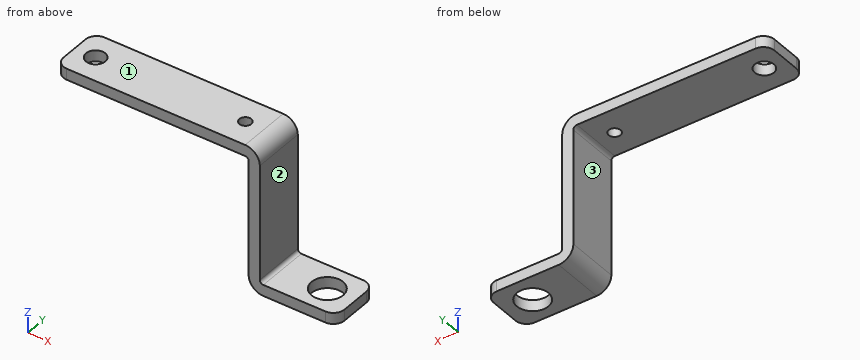
```python
from build123d import *

# Parameters (mm, degrees)
BASE_FLANGE1_DEPTH   = 3.175
EDGE_FLANGE1_DEPTH   = 15
EDGE_FLANGE2_DEPTH   = 15
M5_CLEARANCE_HOLE1_D = 5.5
M8_CLEARANCE_HOLE1_D = 9
FILLET1_R            = 3.175
M3_CLEARANCE_HOLE1_D = 3.4


# Sheet-metal steps are written as plain solids
with BuildPart() as part:
    # Sketch2 → Base-Flange1 (new body)
    with BuildSketch(Plane.XY):
        Polygon((79.909284585, 306.128054742), (73.909284585, 306.128054742), (73.909284585, 321.128054742), (79.909284585, 321.128054742), (127.909284585, 321.128054742), (127.909284585, 306.128054742), align=None)
    extrude(amount=BASE_FLANGE1_DEPTH)

    # Edge-Flange1 section (across the edge) → Edge-Flange1 (add)
    with BuildSketch(Plane(origin=(128.909284585, 321.128054742, 0), x_dir=(-1, 0, 0), z_dir=(0, -1, 0))):
        with BuildLine():
            Line((-3.175, 1), (-3.175, 33.738))
            Line((-3.175, 33.738), (0, 33.738))
            Line((0, 33.738), (0, 1))
            ThreePointArc((0, 1), (0.292893219, 0.292893219), (1, 0))
            Line((1, 0), (1, -3.175))
            ThreePointArc((1, -3.175), (-1.952170811, -1.952170811), (-3.175, 1))
        make_face()
    extrude(amount=EDGE_FLANGE1_DEPTH)

    # Edge-Flange2 section (across the edge) → Edge-Flange2 (add)
    with BuildSketch(Plane(origin=(132.084284585, 306.128054742, -34.738), x_dir=(0, 0, 1), z_dir=(0, 1, 0))):
        with BuildLine():
            Line((-3.175, 1), (-3.175, 21.825))
            Line((-3.175, 21.825), (0, 21.825))
            Line((0, 21.825), (0, 1))
            ThreePointArc((0, 1), (0.292893219, 0.292893219), (1, 0))
            Line((1, 0), (1, -3.175))
            ThreePointArc((1, -3.175), (-1.952170811, -1.952170811), (-3.175, 1))
        make_face()
    extrude(amount=EDGE_FLANGE2_DEPTH)

    # M5 Clearance Hole1 (through all)
    with Locations(Plane.XY.offset(3.175)):
        with Locations((79.909284585, 313.628054742)):
            Hole(M5_CLEARANCE_HOLE1_D / 2)

    # M8 Clearance Hole1 (through all)
    with Locations(Plane.XY.offset(-34.738)):
        with Locations((145.909284585, 313.628054742)):
            Hole(M8_CLEARANCE_HOLE1_D / 2)

    # Fillet1
    fillet1_edges = [part.edges().sort_by_distance(p)[0] for p in [
        (73.909284585, 306.128054742, 1.5875),
        (73.909284585, 321.128054742, 1.5875),
        (153.909284585, 306.128054742, -36.3255),
        (153.909284585, 321.128054742, -36.3255),
    ]]
    fillet(fillet1_edges, radius=FILLET1_R)

    # M3 Clearance Hole1 (through all)
    with Locations(Plane.XY.offset(3.175)):
        with Locations((122.609284585, 313.578054742)):
            Hole(M3_CLEARANCE_HOLE1_D / 2)


solid = part.part
```
The model under review builds one solid part; all positions refer to its coordinate system, in mm. Face numbers are marked on the shaded views. A direction names the side the tool comes from. Round coordinates to 2 decimals unless told otherwise and drop trailing zeros. Write each loop counter-clockwise with the first axis right and the second up, starting at its lowest first coordinate (ties: lowest second). Pieces come first, ordered by that corner, then holes. Notation, with made-up numbers: (-13, 88.25) -> (9, 88.25) arc R30 cw to (9, 122.25) -> close; hole circle Ø6 at (68, -38.5). An arc over 180 degrees is marked (long way). Use CSV: the item, a comma, the result in double quotes.
Q1. Consider section A-A (x = 148). Give the boundary of the cut face in (y, z), then the cut area to 3 significant figures.
Checks:
outline,"(306.13, -37.91) -> (309.64, -37.91) -> (309.64, -34.74) -> (306.13, -34.74) -> close; (317.61, -37.91) -> (321.13, -37.91) -> (321.13, -34.74) -> (317.61, -34.74) -> close"
area,"22.3 mm²"
Q2. Consider section B-B (y = 308). Give the boundary of the cut face in (x, z) (3 decimals), then the cut area to 3 significant figures.
Checks:
outline,"(74.189, 0) -> (127.909, 0) arc R1 cw to (128.909, -1) -> (128.909, -33.738) arc R4.175 ccw to (133.084, -37.913) -> (153.63, -37.913) -> (153.63, -34.738) -> (133.084, -34.738) arc R1 cw to (132.084, -33.738) -> (132.084, -1) arc R4.175 ccw to (127.909, 3.175) -> (74.189, 3.175) -> close"
area,"366 mm²"
Q3. For pin 1 Ø2 at (x, y) = (96.5, 311.5) entering from -Z; pin 2 Ø4.5 at (y, z) = (315, -17.5) entering from +X; pin 3 Ø1.5 at (y, z) = (310, -19.5) entering from -X; pin 4 Ø4.5 at (x, y) = (79.91, 313.63) entering from +Z, all flat-tipped, find the tip position at first contact; note any pin that passes through.
Checks:
pin 1,"z = 0"
pin 2,"x = 132.08"
pin 3,"x = 128.91"
pin 4,"through"
Q4. For the marked faces 1, 2 and 3, list the 3-axis set-ups (+Z, -Z, +X, -X, +Y, -Y) from which the entire face can be reached by the end or side of a thin tool; tool diameter is ignored.
Checks:
face 1,"+Z, +X, -X, +Y, -Y"
face 2,"+Z, +X, +Y, -Y"
face 3,"-Z, -X, +Y, -Y"
Q5. Consider section C-C (z = -30.5). Give the boundary of the cut face in (x, y).
Checks:
outline,"(128.91, 306.13) -> (132.08, 306.13) -> (132.08, 321.13) -> (128.91, 321.13) -> close"
Q6. Consider section D-D (x = 138.5). Give the boundary of the cut face in (y, z).
Checks:
outline,"(306.13, -37.91) -> (321.13, -37.91) -> (321.13, -34.74) -> (306.13, -34.74) -> close"
Q7. To check wall thickness, follow probe 1 along X at (y, z) = (307.75, -30); probe 2 along Z at (x, y) = (89, 309.5) (3 decimals); probe 3 along Z at (x, y) = (150.5, 317.25). State the ranges of each line that lie inside material, in increasing order. Write a range as [from, to].
Checks:
probe 1,"[128.91, 132.08]"
probe 2,"[0, 3.175]"
probe 3,"[-37.91, -34.74]"
